```python
from build123d import *

# Parameters (mm, degrees)
SKETCH1_R           = 1.5
BOSS_EXTRUDE1_DEPTH = 1.5
SKETCH3_W           = 3
SKETCH3_H           = 12
CUT_EXTRUDE1_DEPTH  = 2
BOSS_EXTRUDE3_DEPTH = 5


with BuildPart() as part:
    # Sketch1 → Boss-Extrude1 (new body)
    with BuildSketch(Plane(origin=(0, 0, 0), x_dir=(1, 0, 0), z_dir=(0, 1, 0))):
        Polygon((-21, 11.5), (-21, 17), (-17, 21), (17, 21), (21, 17), (21, 11.5), (21, -11.5), (21, -17), (17, -21), (-17, -21), (-21, -17), (-21, -11.5), align=None)
        with Locations(Location((-15.5, 15.5, 0), (0, 0, 270))):
            Circle(SKETCH1_R, mode=Mode.SUBTRACT)
        with Locations(Location((15.5, 15.5, 0), (0, 0, 270))):
            Circle(SKETCH1_R, mode=Mode.SUBTRACT)
        with Locations(Location((15.5, -15.5, 0), (0, 0, 90))):
            Circle(SKETCH1_R, mode=Mode.SUBTRACT)
        with Locations(Location((-15.5, -15.5, 0), (0, 0, 90))):
            Circle(SKETCH1_R, mode=Mode.SUBTRACT)
        with Locations(Location((-8.5, 8.5, 0), (0, 0, 270))):
            Circle(SKETCH1_R, mode=Mode.SUBTRACT)
        with Locations(Location((8.5, 8.5, 0), (0, 0, 270))):
            Circle(SKETCH1_R, mode=Mode.SUBTRACT)
        with Locations(Location((8.5, -8.5, 0), (0, 0, 90))):
            Circle(SKETCH1_R, mode=Mode.SUBTRACT)
        with Locations(Location((-8.5, -8.5, 0), (0, 0, 90))):
            Circle(SKETCH1_R, mode=Mode.SUBTRACT)
    extrude(amount=BOSS_EXTRUDE1_DEPTH)

    # Sketch3 → Cut-Extrude1 (cut)
    with BuildSketch(Plane.XZ):
        with Locations((6.5, 0)):
            Rectangle(SKETCH3_W, SKETCH3_H)
        with Locations((-6.5, 0)):
            Rectangle(SKETCH3_W, SKETCH3_H)
    extrude(amount=-CUT_EXTRUDE1_DEPTH, mode=Mode.SUBTRACT)

    # Sketch2 → Boss-Extrude3 (add)
    with BuildSketch(Plane(origin=(0, 1.5, 0), x_dir=(1, 0, 0), z_dir=(0, 1, 0))):
        Polygon((17, 21), (14.171572875, 21), (15.585786438, 19.585786438), (19.585786438, 15.585786438), (21, 14.171572875), (21, 17), align=None)
        Polygon((-17, 21), (-21, 17), (-21, 14.171572875), (-19.585786438, 15.585786438), (-15.585786438, 19.585786438), (-14.171572875, 21), align=None)
        Polygon((-19.585786438, -15.585786438), (-21, -14.171572875), (-21, -17), (-17, -21), (-14.171572875, -21), (-15.585786438, -19.585786438), align=None)
        Polygon((21, -14.171572875), (14.171572875, -21), (17, -21), (21, -17), align=None)
    extrude(amount=BOSS_EXTRUDE3_DEPTH)


solid = part.part
```
Check sheet for the modelled part. Datum: model origin and axes. Units: mm. A direction names the side the tool comes from. Give positions to 0.01 mm unless a question says otherwise; leave off trailing zeros. Order: outer loops, then holes, each group sorted by start corner. A loop starts at its lowest first (then second) coordinate and runs counter-clockwise, first axis right, second up. Notation, with made-up numbers: M 64.25,40.25 L 91.25,40.25 A27 cw 91.25,75.25 Z; hole C 36.5,35.5 d6. An arc over 180 degrees is marked long. Answer in a Markdown table with one row per item. Add a question column.
Q1. Thickness scan on L1, parallel to X at y = 0.35, z = 15.5; L2, parallel to X at y = 1, z = 8.5; L3, parallel to Y at x = 18.5, z = 13.5. Record the ranges inside material, lowest first.
Q2. Sectioned sample at A-A, the plane x = 8.5. Record the boundary of the cut face in (y, z), and give its area (3 significant figures).
Q3. Sectioned sample at C-C, the plane z = 8.5. Record the boundary of the cut face in (x, y), and give its area (3 significant figures).
Q4. Release check for a two-part mould opening along Z. For faces 4 (the flat face through (-19, 3, -19)), 5 (the flat face through (-21, 1, 0)), 6 (the cylindrical face through (-15.43, 0.74, -17)) record: released by +Z, released by -Z, zero draft, split by the parting line, or undercut.
Q5. Sectioned sample at D-D, the plane y = 5.75. Record the boundary of the cut face in (x, z), and give its area (3 significant figures).
Q6. Gauge pin test, flat end, axial feed: pin 1 Ø21 at (x, z) = (-4, 9) entering from +Y. Record the tip position at first contact, or that the pin passes through.
Q7. Access from +Z, -Z, +X, -X, +Y, -Y to the whole of each face (thin tool, end or side, straight path). Record for faces 1 (the flat face through (19, 3, -19)), 2 (the flat face through (0, 1.5, 0)), 3 (the flat face through (5, 1, 0)).
Q8. Sectioned sample at B-B, the plane x = -6. Record the boundary of the cut face in (y, z), and give its area (3 significant figures).
Verdict:
| question | item | result |
|---|---|---|
| 1 | L1 | -21 to -17, -14 to 14, 17 to 21 |
| 1 | L2 | -21 to -10, -7 to 7, 10 to 21 |
| 1 | L3 | 0 to 1.5 |
| 2 | outline | M 0,-21 L 1.5,-21 L 1.5,-10 L 0,-10 Z; M 0,-7 L 1.5,-7 L 1.5,7 L 0,7 Z; M 0,10 L 1.5,10 L 1.5,21 L 0,21 Z |
| 2 | area | 54.0 mm² |
| 3 | outline | M -21,0 L -10,0 L -10,1.5 L -21,1.5 Z; M -7,0 L 7,0 L 7,1.5 L -7,1.5 Z; M 10,0 L 21,0 L 21,1.5 L 10,1.5 Z |
| 3 | area | 54.0 mm² |
| 4 | face 4 | released by -Z |
| 4 | face 5 | zero draft |
| 4 | face 6 | undercut |
| 5 | outline | M -21,-17 L -17,-21 L -14.17,-21 L -21,-14.17 Z; M -21,14.17 L -14.17,21 L -17,21 L -21,17 Z; M 14.17,-21 L 17,-21 L 21,-17 L 21,-14.17 Z; M 14.17,21 L 21,14.17 L 21,17 L 17,21 Z |
| 5 | area | 61.3 mm² |
| 6 | pin 1 | y = 1.5 |
| 7 | face 1 | -Z, +X, +Y, -Y |
| 7 | face 2 | +Y |
| 7 | face 3 | +Y, -Y |
| 8 | outline | M 0,-21 L 1.5,-21 L 1.5,-6 L 0,-6 Z; M 0,6 L 1.5,6 L 1.5,21 L 0,21 Z |
| 8 | area | 45.0 mm² |
